Design review of the part built by this model. Coordinates are the model's own, in mm. A direction names the side the tool comes from. Give positions to 0.01 mm unless a question says otherwise; leave off trailing zeros. Order: outer loops, then holes, each group sorted by start corner. A loop starts at its lowest first (then second) coordinate and runs counter-clockwise, first axis right, second up. Notation, with made-up numbers: (-39.75, 56) -> (13.25, 56) arc R11 ccw to (13.25, 63) -> close; hole circle Ø3 at (-22, -24). An arc over 180 degrees is marked (long way). Use a Markdown table: item, result. Add a question column.
```python
from build123d import *

# Parameters (mm, degrees)
SKETCH1_R           = 2.85
BOSS_EXTRUDE1_DEPTH = 3
SKETCH2_R           = 1.5
BOSS_EXTRUDE2_DEPTH = 16
CHAMFER1_SIZE       = 0.3
CUT_EXTRUDE1_DEPTH  = 2


with BuildPart() as part:
    # Sketch1 → Boss-Extrude1 (new body)
    with BuildSketch(Plane.XY):
        Circle(SKETCH1_R)
    extrude(amount=BOSS_EXTRUDE1_DEPTH)

    # Sketch2 → Boss-Extrude2 (add)
    with BuildSketch(Plane(origin=(0, 0, 0), x_dir=(-1, 0, 0), z_dir=(0, 0, -1))):
        Circle(SKETCH2_R)
    extrude(amount=BOSS_EXTRUDE2_DEPTH)

    # Chamfer1
    chamfer1_edges = [part.edges().sort_by_distance(p)[0] for p in [
        (1.5, 0, -16),
    ]]
    chamfer(chamfer1_edges, length=CHAMFER1_SIZE)

    # Sketch3 → Cut-Extrude1 (cut)
    with BuildSketch(Plane.XY.offset(3)):
        Polygon((0, 1.443375673), (-1.25, 0.721687836), (-1.25, -0.721687836), (0, -1.443375673), (1.25, -0.721687836), (1.25, 0.721687836), align=None)
    extrude(amount=-CUT_EXTRUDE1_DEPTH, mode=Mode.SUBTRACT)


solid = part.part
```
1) Machinability: for faces 1 (the flat face through (1.2, -1.2, 0)), 2 (the flat face through (0.616, -1.088, 2.014)), 3 (the cylindrical face through (-2.262, -1.734, 1.479)), which of the approach directions +Z, -Z, +X, -X, +Y, -Y give a long, thin tool a straight path to every point of the face, cutting with its end or side? Answer none if there is none.
2) Add section C-C (z = -10.75). Give the boundary of the cut face in (x, y), then the cut area to 3 significant figures.
3) Add section B-B (y = 0). Give the boundary of the cut face in (x, z), then the cut area to 3 significant figures.
4) Insertion check: pin 1 (1.2 mm diameter, centred on x = -0.5, y = 0, fed in from +Z). The pin has a flat end and moves straight along its axis. Give the tip position at first contact, or say it passes through.
5) Add section D-D (x = -2.4). Give the boundary of the cut face in (y, z).
6) Add section A-A (z = 2). Give the boundary of the cut face in (x, y), then the cut area to 3 significant figures.
7) For L1, parallel to Y at x = -0.4, z = 1.5; L2, parallel to Z at x = -0.5, y = 1.9; L3, parallel to Z at x = -0.6, y = 0.55, list the stretches that pass through material, from the lowest coordinate up. Write a range as [from, to].
Worked answers:
| question | item | result |
|---|---|---|
| 1 | face 1 | -Z |
| 1 | face 2 | +Z |
| 1 | face 3 | +Z, -Z |
| 2 | outline | circle Ø3 at (0, 0) |
| 2 | area | 7.07 mm^2 |
| 3 | outline | (-2.85, 0) -> (-1.5, 0) -> (-1.5, -15.7) -> (-1.2, -16) -> (1.2, -16) -> (1.5, -15.7) -> (1.5, 0) -> (2.85, 0) -> (2.85, 3) -> (1.25, 3) -> (1.25, 1) -> (-1.25, 1) -> (-1.25, 3) -> (-2.85, 3) -> close |
| 3 | area | 60.0 mm^2 |
| 4 | pin 1 | z = 1 |
| 5 | outline | (-1.54, 0) -> (1.54, 0) -> (1.54, 3) -> (-1.54, 3) -> close |
| 6 | outline | circle Ø5.7 at (0, 0); hole (-1.25, -0.72) -> (0, -1.44) -> (1.25, -0.72) -> (1.25, 0.72) -> (0, 1.44) -> (-1.25, 0.72) -> close |
| 6 | area | 20.1 mm^2 |
| 7 | L1 | [-2.82, -1.21], [1.21, 2.82] |
| 7 | L2 | [0, 3] |
| 7 | L3 | [-16, 1] |
